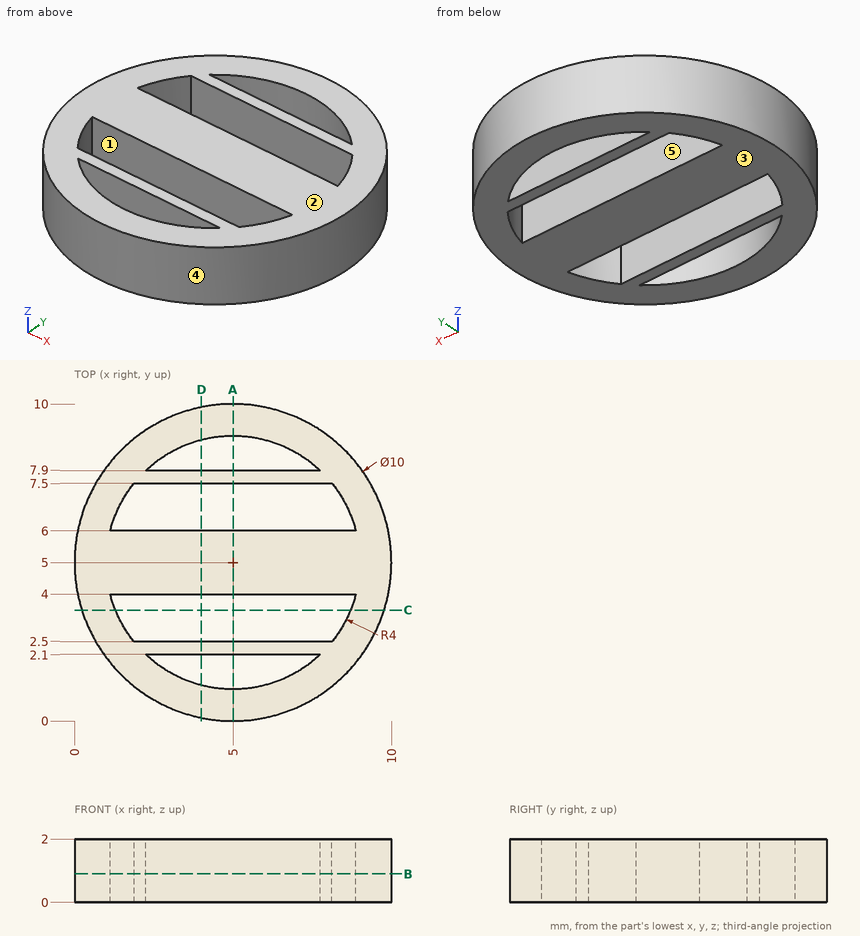
Study the drawing (mm; zero at the part's minimum x, y, z) and answer. A direction names the side the tool comes from. Coordinates: 2 decimals unless noted, no trailing zeros. Order: outer loops, then holes, each group sorted by start corner. A loop starts at its lowest first (then second) coordinate and runs counter-clockwise, first axis right, second up. Notation, with made-up numbers: M 35,-28.5 L 63,-28.5 A30 ccw 63,2.5 Z; hole C 66,19 d2. An arc over 180 degrees is marked long. Use CSV: the item, a comma, the result in double quotes.
Q1. Section D-D (x = 4) is taken. Determine the outline of the cut face in (y, z), then the cut area to 3 significant figures.
Here are the results:
outline,"M 0.1,0 L 1.13,0 L 1.13,2 L 0.1,2 Z; M 2.1,0 L 2.5,0 L 2.5,2 L 2.1,2 Z; M 4,0 L 6,0 L 6,2 L 4,2 Z; M 7.5,0 L 7.9,0 L 7.9,2 L 7.5,2 Z; M 8.87,0 L 9.9,0 L 9.9,2 L 8.87,2 Z"
area,"9.70 mm2"
Q2. Straight lines are drawn through the part: L1, parallel to Y at x = 5, z = 0.65; L2, parallel to Y at x = 7, z = 0.25; L3, parallel to Y at x = 1.75, z = 0.5. For each, find the intervals that lie inside material, in ascending order.
Here are the results:
L1,"0 to 1, 2.1 to 2.5, 4 to 6, 7.5 to 7.9, 9 to 10"
L2,"0.42 to 1.54, 2.1 to 2.5, 4 to 6, 7.5 to 7.9, 8.46 to 9.58"
L3,"1.2 to 2.67, 4 to 6, 7.33 to 8.8"
Q3. Section A-A (x = 5) is taken. Determine the outline of the cut face in (y, z), then the cut area to 3 significant figures.
Here are the results:
outline,"M 0,0 L 1,0 L 1,2 L 0,2 Z; M 2.1,0 L 2.5,0 L 2.5,2 L 2.1,2 Z; M 4,0 L 6,0 L 6,2 L 4,2 Z; M 7.5,0 L 7.9,0 L 7.9,2 L 7.5,2 Z; M 9,0 L 10,0 L 10,2 L 9,2 Z"
area,"9.60 mm2"
Q4. Given pin 1 Ø1 at (x, z) = (4, 1.5) entering from -Y; pin 2 Ø0.6 at (x, z) = (5.5, 1) entering from +Y, each flat-ended and moving along its own axis, determine where each tip first touches the part or whether it passes through.
Here are the results:
pin 1,"y = 0.03"
pin 2,"y = 10"
Q5. Section C-C (y = 3.5) is taken. Determine the outline of the cut face in (x, z), then the cut area to 3 significant figures.
Here are the results:
outline,"M 0.23,0 L 1.29,0 L 1.29,2 L 0.23,2 Z; M 8.71,0 L 9.77,0 L 9.77,2 L 8.71,2 Z"
area,"4.25 mm2"
Q6. Section B-B (z = 0.9) is taken. Determine the outline of the cut face in (x, y) (1 decimal).
Here are the results:
outline,"C 5,5 d10; hole M 1.1,4 A4 ccw 1.9,2.5 L 8.1,2.5 A4 ccw 8.9,4 Z; hole M 1.1,6 L 8.9,6 A4 ccw 8.1,7.5 L 1.9,7.5 A4 ccw Z; hole M 2.2,2.1 A4 ccw 7.8,2.1 Z; hole M 2.2,7.9 L 7.8,7.9 A4 ccw Z"
Q7. A tool of negligible diameter and unlimited length cuts with its end or side. For the marked faces 1 and 2, from which of +Z, -Z, +X, -X, +Y, -Y can it reach the whole face along a straight path? Write none if from no direction.
Here are the results:
face 1,"+Z, -Z"
face 2,"+Z, +X, -X, +Y, -Y"
Q8. Determine the mould class of the marked faces 3, 4 and 5 for opening direction Y: pulls with the +Y half, pulls with the -Y half, needs draft (parallel to the pull), parting line crosses it, or undercut.
Here are the results:
face 3,"needs draft"
face 4,"parting line crosses it"
face 5,"undercut"
